from build123d import *

# Parameters (mm, degrees)
SKETCH1_W                       = 1676.4
SKETCH1_H                       = 101.6
BOSS_EXTRUDE1_DEPTH             = 101.6
SKETCH3_W                       = 76.2
SKETCH3_H                       = 76.2
CUT_EXTRUDE1_DEPTH              = 127
SKETCH5_W                       = 76.2
SKETCH5_H                       = 76.2
BOSS_EXTRUDE2_DEPTH             = 114.3
SKETCH6_W                       = 76.2
SKETCH6_H                       = 12.7
BOSS_EXTRUDE3_DEPTH             = 152.4
BOSS_EXTRUDE4_REACH             = 52.8
SKETCH7_R                       = 12.7
BOSS_EXTRUDE4_DIRECTION_2_REACH = 52.8
SKETCH8_R                       = 76.2
BOSS_EXTRUDE5_DEPTH             = 12.7
BOSS_EXTRUDE5_DEPTH_BACK        = 12.7
SKETCH9_R                       = 6.35
CUT_EXTRUDE2_DEPTH              = 12.7


with BuildPart() as part:
    # Sketch1 → Boss-Extrude1 (new body)
    with BuildSketch(Plane.XY):
        with Locations((838.2, 50.8)):
            Rectangle(SKETCH1_W, SKETCH1_H)
    extrude(amount=BOSS_EXTRUDE1_DEPTH)

    # Sketch3 → Cut-Extrude1 (cut)
    with BuildSketch(Plane.ZY):
        with Locations((50.8, 50.8)):
            Rectangle(SKETCH3_W, SKETCH3_H)
    extrude(amount=-CUT_EXTRUDE1_DEPTH, mode=Mode.SUBTRACT)

    # Sketch5 → Boss-Extrude2 (add)
    with BuildSketch(Plane(origin=(0, 101.6, 0), x_dir=(1, 0, 0), z_dir=(0, 1, 0))):
        with Locations((1625.6, -50.8)):
            Rectangle(SKETCH5_W, SKETCH5_H)
    extrude(amount=BOSS_EXTRUDE2_DEPTH)

    # Sketch6 → Boss-Extrude3 (add)
    with BuildSketch(Plane(origin=(0, 215.9, 0), x_dir=(1, 0, 0), z_dir=(0, 1, 0))):
        with Locations((1625.6, -19.05)):
            Rectangle(SKETCH6_W, SKETCH6_H)
        with Locations((1625.6, -82.55)):
            Rectangle(SKETCH6_W, SKETCH6_H)
    extrude(amount=BOSS_EXTRUDE3_DEPTH)

    # Boss-Extrude4: up to this face of the body (flat: up to its plane)
    boss_extrude4_end = Plane(part.part.faces().sort_by_distance((1625.6, 292.1, 25.4))[0])
    # Sketch7 → Boss-Extrude4 (add, up to the picked face)
    with BuildSketch(Plane(origin=(0, 0, 50.8), x_dir=(-1, 0, 0), z_dir=(0, 0, -1)), mode=Mode.PRIVATE) as boss_extrude4_sk1:
        with Locations((-1625.6, 311.15)):
            Circle(SKETCH7_R)
    boss_extrude4_tool1 = split(extrude(boss_extrude4_sk1.sketch, amount=BOSS_EXTRUDE4_REACH, mode=Mode.PRIVATE), bisect_by=boss_extrude4_end, keep=Keep.BOTH, mode=Mode.PRIVATE)
    add(boss_extrude4_tool1.solids().sort_by_distance((1625.6, 311.15, 50.8))[0])

    # Boss-Extrude4 direction 2: up to this face of the body (flat: up to its plane)
    boss_extrude4_direction_2_end = Plane(part.part.faces().sort_by_distance((1625.6, 292.1, 76.2))[0])
    # Sketch7 → Boss-Extrude4 direction 2 (add, up to the picked face)
    with BuildSketch(Plane(origin=(0, 0, 50.8), x_dir=(-1, 0, 0), z_dir=(0, 0, -1)), mode=Mode.PRIVATE) as boss_extrude4_direction_2_sk1:
        with Locations((-1625.6, 311.15)):
            Circle(SKETCH7_R)
    boss_extrude4_direction_2_tool1 = split(extrude(boss_extrude4_direction_2_sk1.sketch, amount=-BOSS_EXTRUDE4_DIRECTION_2_REACH, mode=Mode.PRIVATE), bisect_by=boss_extrude4_direction_2_end, keep=Keep.BOTH, mode=Mode.PRIVATE)
    add(boss_extrude4_direction_2_tool1.solids().sort_by_distance((1625.6, 311.15, 50.8))[0])

    # Sketch8 → Boss-Extrude5 (add, two sides)
    with BuildSketch(Plane(origin=(0, 0, 50.8), x_dir=(-1, 0, 0), z_dir=(0, 0, -1))) as boss_extrude5_sk:
        with Locations((-1625.6, 311.15)):
            Circle(SKETCH8_R)
    extrude(amount=BOSS_EXTRUDE5_DEPTH)
    extrude(boss_extrude5_sk.sketch, amount=-BOSS_EXTRUDE5_DEPTH_BACK)

    # Sketch9 → Cut-Extrude2 (cut)
    with BuildSketch(Plane(origin=(0, 101.6, 0), x_dir=(1, 0, 0), z_dir=(0, 1, 0))):
        with Locations((38.1, -50.8)):
            Circle(SKETCH9_R)
        with Locations((1524, -50.8)):
            Circle(SKETCH9_R)
    extrude(amount=-CUT_EXTRUDE2_DEPTH, mode=Mode.SUBTRACT)


solid = part.part
Design review of the part built by this model. Coordinates are the model's own, in mm. A direction names the side the tool comes from. Round coordinates to 2 decimals unless told otherwise and drop trailing zeros. Loops run counter-clockwise (first coordinate to the right, second up) from the corner with the lowest first, then second, coordinate; pieces in that order, holes last. Notation, with made-up numbers: M 23,44.5 L 61,44.5 A19 cw 61,73.5 Z; hole C 27,56 d5. An arc over 180 degrees is marked long. Answer as a JSON object with one key per item and string values.
Item 1: We need section D-D on y = 178. Give the boundary of the cut face in (x, z), and give its area (3 significant figures).
Answer sheet:
{"outline": "M 1587.5,12.7 L 1663.7,12.7 L 1663.7,88.9 L 1587.5,88.9 Z", "area": "5,810 mm^2"}
Item 2: The part is to be moulded in two halves that separate along Z. For faces 6 (the flat face through (63, 50, 88.9)), 7 (the flat face through (1663.7, 203, 51)), 8 (the flat face through (1625, 215.9, 50)), 9 (the flat face through (1625, 233, 88.9)), say which applies: pulls with the +Z half, pulls with the -Z half, needs draft (parallel to the pull), parting line crosses it, or undercut.
Answer sheet:
{"face 6": "undercut", "face 7": "needs draft", "face 8": "undercut", "face 9": "pulls with the +Z half"}
Item 3: We need section C-C on y = 279. Give the boundary of the cut face in (x, z), and give its area (3 significant figures).
Answer sheet:
{"outline": "M 1556.51,38.1 L 1694.69,38.1 L 1694.69,63.5 L 1556.51,63.5 Z; M 1587.5,12.7 L 1663.7,12.7 L 1663.7,25.4 L 1587.5,25.4 Z; M 1587.5,76.2 L 1663.7,76.2 L 1663.7,88.9 L 1587.5,88.9 Z", "area": "5,450 mm^2"}
Item 4: Clearance check with flat-ended pins moving along their axes: P1, Ø23, axis at y = 35, z = 63.5, coming from the -X side; P2, Ø23, axis at y = 206, z = 54, coming from the -X side; P3, Ø1, axis at x = 654, z = 57.5, coming from the -Y side; P4, Ø14, axis at x = 1607.5, z = 82.5, coming from the +Y side. State where each tip first meets the part, or that it passes through.
Answer sheet:
{"P1": "stops at x = 127", "P2": "stops at x = 1587.5", "P3": "stops at y = 0", "P4": "stops at y = 368.3"}
Item 5: We need section B-B on y = 349. Give the boundary of the cut face in (x, z).
Answer sheet:
{"outline": "M 1559.47,38.1 L 1691.73,38.1 L 1691.73,63.5 L 1559.47,63.5 Z; M 1587.5,12.7 L 1663.7,12.7 L 1663.7,25.4 L 1587.5,25.4 Z; M 1587.5,76.2 L 1663.7,76.2 L 1663.7,88.9 L 1587.5,88.9 Z"}
Item 6: Wall thickness on L1, parallel to X at y = 93, z = 50.8; L2, parallel to Y at x = 69.5, z = 54; L3, parallel to X at y = 97, z = 54: over which ranges is each line inside the solid? List them lowest first. Write a range as from..to.
Answer sheet:
{"L1": "x = 0..31.75, 44.45..1517.65, 1530.35..1676.4", "L2": "y = 0..12.7, 88.9..101.6", "L3": "x = 0..32.62, 43.58..1518.52, 1529.48..1676.4"}
Item 7: We need section A-A on y = 56.5. Give the boundary of the cut face in (x, z).
Answer sheet:
{"outline": "M 0,0 L 1676.4,0 L 1676.4,101.6 L 0,101.6 L 0,88.9 L 127,88.9 L 127,12.7 L 0,12.7 Z"}
Item 8: Machinability: for faces 1 (the flat face through (826, 52, 0)), 2 (the flat face through (63, 12.7, 50)), 3 (the flat face through (826, 0, 50)), 4 (the cylindrical face through (1552.92, 334.04, 50.62)), 5 (the flat face through (1676.4, 50, 50)), which of the approach directions +Z, -Z, +X, -X, +Y, -Y give a long, thin tool a straight path to every point of the face, cutting with its end or side? Answer none if there is none.
Answer sheet:
{"face 1": "-Z, +X, -X, +Y, -Y", "face 2": "-X", "face 3": "+Z, -Z, +X, -X, -Y", "face 4": "none", "face 5": "+Z, -Z, +X, -Y"}
